Source: CAD feature listing. Evaluate the final solid. Frame: model axes, mm. A direction names the side the tool comes from. Coordinates: 2 decimals unless noted, no trailing zeros. Write each loop counter-clockwise with the first axis right and the second up, starting at its lowest first coordinate (ties: lowest second). Pieces come first, ordered by that corner, then holes. Notation, with made-up numbers: (-35.5, -13) -> (-17.5, -13) arc R19 cw to (-17.5, 12) -> close; hole circle Ø5 at (4, 8.5). An arc over 180 degrees is marked (long way). One line per item, written item: value. Start each with the question number.
1. Section query A-A, the plane x = 0. Output: boundary loops of the cut face in (y, z) (3 decimals).
2. Line query: line 1 (Y direction, x = 0, z = 9) (3 decimals); line 2 (X direction, y = -15, z = 5.75); line 3 (Y direction, x = 4, z = 4.25). Output: solid intervals per line, ascending.
3. Mould query, pull axis Z, two halves, no side actions, for faces 6 (the flat face through (-2, -19, 9.525)), 7 (the cylindrical face through (12.242, -21.869, 4.122)), 8 (the flat face through (-21.304, 8.22, 4.696)), 9 (the cylindrical face through (-24.29, -3.03, 3.59)). Classes: released by +Z, released by -Z, zero draft, split by the parting line, or undercut.
4. Access query for faces 1 (the flat face through (16.739, -19, 5)), 2 (the flat face through (13, -18.65, 5)), 3 (the flat face through (-2, -19, 0)), 4 (the cylindrical face through (-21.675, 0.014, 4.696)), 5 (the flat face through (-16.739, -19, 5)). Directions: +Z, -Z, +X, -X, +Y, -Y. A direction counts if a zero-diameter tool reaches every point of the face in a straight line with its end or side. Return the directions, or none.
5. First-contact query: P1, Ø4, axis at x = -5, y = -14, coming from the -Z side; P2, Ø3.5, axis at x = -22.5, z = 3.5, coming from the +Y side; P3, Ø1.5, axis at x = -24, z = 4, coming from the -Y side. Flat tips, straight axial feed; report the tip coordinate or a pass-through.
6. Section query D-D, the plane z = 8. Output: boundary loops of the cut face in (x, y) (3 decimals), and give its area (3 significant figures).
7. Section query C-C, the plane y = 0. Output: boundary loops of the cut face in (x, z) (3 decimals), and give its area (3 significant figures).
8. Section query B-B, the plane z = 4. State how many separate pieces and enclosed holes the cut face has, and give its area (3 significant figures).
from build123d import *

# Parameters (mm, degrees)
SKETCH1_R           = 18.5
BOSS_EXTRUDE1_DEPTH = 9.525
SKETCH2_R           = 1.3890625
CUT_EXTRUDE1_DEPTH  = 6.35
CUT_EXTRUDE2_REACH  = 40.448
SKETCH3_R           = 1.3890625


with BuildPart() as part:
    # Sketch1 → Boss-Extrude1 (new body)
    with BuildSketch(Plane.XY):
        with BuildLine():
            Line((-16.7386, 13.770435543), (-26, 2.512776367))
            Line((-26, 2.512776367), (-26, 1))
            Line((-26, 1), (-21.651919661, 1))
            ThreePointArc((-21.651919661, 1), (-21.675, 0), (-21.651919661, -1))
            Line((-21.651919661, -1), (-26, -1))
            Line((-26, -1), (-26, -5))
            Line((-26, -5), (-21.090415477, -5))
            ThreePointArc((-21.090415477, -5), (-19.416197823, -9.634152122), (-16.7386, -13.770435543))
            Line((-16.7386, -13.770435543), (-16.7386, -25))
            Line((-16.7386, -25), (16.7386, -25))
            Line((16.7386, -25), (16.7386, -13.770435543))
            ThreePointArc((16.7386, -13.770435543), (13.770435543, 16.7386), (-16.7386, 13.770435543))
        make_face()
        with Locations(Location((0, 0, 0), (0, 0, 180))):
            Circle(SKETCH1_R, mode=Mode.SUBTRACT)
    extrude(amount=BOSS_EXTRUDE1_DEPTH)

    # Sketch2 → Cut-Extrude1 (cut)
    with BuildSketch(Plane.XZ.offset(25)):
        with Locations(Location((-13.4747, 4.7625, 0), (0, 0, 270))):
            Circle(SKETCH2_R)
        with Locations(Location((13.4747, 4.7625, 0), (0, 0, 270))):
            Circle(SKETCH2_R)
    extrude(amount=-CUT_EXTRUDE1_DEPTH, mode=Mode.SUBTRACT)

    # Cut-Extrude2: up to this plane
    cut_extrude2_end = Plane(origin=(-16.7386, 13.770435543, 9.525), z_dir=(0.7722537485582471, -0.635314211896551, 0))
    # Sketch3 → Cut-Extrude2 (cut, up to the surface)
    with BuildSketch(Plane.XZ.offset(5), mode=Mode.PRIVATE) as cut_extrude2_sk1:
        with Locations(Location((-23.545207739, 4.7625, 0), (0, 0, 180))):
            Circle(SKETCH3_R)
    cut_extrude2_tool1 = split(extrude(cut_extrude2_sk1.sketch, amount=-CUT_EXTRUDE2_REACH, mode=Mode.PRIVATE), bisect_by=cut_extrude2_end, keep=Keep.BOTH, mode=Mode.PRIVATE)
    add(cut_extrude2_tool1.solids().sort_by_distance((-23.545208, -5, 4.7625))[0], mode=Mode.SUBTRACT)


solid = part.part
Computed values:
1. outline: (-25, 0) -> (-18.5, 0) -> (-18.5, 9.525) -> (-25, 9.525) -> close; (18.5, 0) -> (21.675, 0) -> (21.675, 9.525) -> (18.5, 9.525) -> close
2. line 1: y = -25 to -18.5, 18.5 to 21.675
2. line 2: x = -16.74 to -10.83, 10.83 to 16.74
2. line 3: y = -25 to -18.06, 18.06 to 21.3
3. face 6: released by +Z
3. face 7: undercut
3. face 8: zero draft
3. face 9: undercut
4. face 1: +Z, -Z, +X, -Y
4. face 2: -Y
4. face 3: -Z, +X, -X, +Y, -Y
4. face 4: +Z, -Z, -X
4. face 5: +Z, -Z, -X, -Y
5. P1: passes through
5. P2: stops at y = 8.89
5. P3: stops at y = -5
6. outline: (-26, -5) -> (-21.09, -5) arc R21.675 ccw to (-16.739, -13.77) -> (-16.739, -25) -> (16.739, -25) -> (16.739, -13.77) arc R21.675 ccw to (-16.739, 13.77) -> (-26, 2.513) -> (-26, 1) -> (-21.652, 1) arc R21.675 ccw to (-21.652, -1) -> (-26, -1) -> close; hole circle Ø37 at (0, 0)
6. area: 635 mm²
7. outline: (-21.675, 0) -> (-18.5, 0) -> (-18.5, 9.525) -> (-21.675, 9.525) -> close; (18.5, 0) -> (21.675, 0) -> (21.675, 9.525) -> (18.5, 9.525) -> close
7. area: 60.5 mm²
8. separate pieces: 3
8. enclosed holes: 1
8. area: 586 mm²
